Check sheet for the modelled part. Datum: model origin and axes. Units: mm. Face numbers are marked on the shaded views. A direction names the side the tool comes from. Round coordinates to 2 decimals unless told otherwise and drop trailing zeros. Write each loop counter-clockwise with the first axis right and the second up, starting at its lowest first coordinate (ties: lowest second). Pieces come first, ordered by that corner, then holes. Notation, with made-up numbers: M 33,77 L 67,77 A18 ccw 67,102 Z; hole C 54.25,74 d1. An arc over 180 degrees is marked long. Answer in a Markdown table with one row per item.
```python
from build123d import *

# Parameters (mm, degrees)
BOSS_EXTRUDE1_DEPTH     = 9
SHELL1_T                = -1
BOSS_EXTRUDE2_DEPTH     = 2
SKETCH3_R               = 6.5
BOSS_EXTRUDE3_DEPTH     = 1.25
SKETCH4_R               = 5
BOSS_EXTRUDE4_DEPTH     = 0.6
CUT_EXTRUDE1_DEPTH      = 26.78996898
CUT_EXTRUDE1_DEPTH_BACK = 26.78996898
SKETCH5_R               = 3.1
BOSS_EXTRUDE5_DEPTH     = 1.8
SKETCH7_W               = 18.24
SKETCH7_H               = 6.5
BOSS_EXTRUDE6_DEPTH     = 2.5
CUT_EXTRUDE2_REACH      = 31.955
SKETCH8_R               = 2.25
FILLET2_R               = 1
CUT_EXTRUDE3_DEPTH      = 30.432125306
CUT_EXTRUDE3_DEPTH_BACK = 1
SKETCH9_R               = 9


with BuildPart() as part:
    # Sketch1 → Boss-Extrude1 (new body)
    with BuildSketch(Plane(origin=(0, 0, 0), x_dir=(1, 0, 0), z_dir=(0, 1, 0))):
        with BuildLine():
            Line((-9.12, 20), (9.12, 20))
            ThreePointArc((9.12, 20), (9.742253967, 19.742253967), (10, 19.12))
            Line((10, 19.12), (10, -19.12))
            ThreePointArc((10, -19.12), (9.742253967, -19.742253967), (9.12, -20))
            Line((9.12, -20), (-9.12, -20))
            ThreePointArc((-9.12, -20), (-9.742253967, -19.742253967), (-10, -19.12))
            Line((-10, -19.12), (-10, 19.12))
            ThreePointArc((-10, 19.12), (-9.742253967, 19.742253967), (-9.12, 20))
        make_face()
    extrude(amount=BOSS_EXTRUDE1_DEPTH)

    # Shell1
    shell1_openings = [part.faces().sort_by_distance(p)[0] for p in [
        (0, 0, 0),
    ]]
    offset(amount=SHELL1_T, openings=shell1_openings, kind=Kind.INTERSECTION)

    # Sketch2 → Boss-Extrude2 (add)
    with BuildSketch(Plane(origin=(0, 9, 0), x_dir=(1, 0, 0), z_dir=(0, 1, 0))):
        with BuildLine():
            Line((9.5, -14), (-9.5, -14))
            Line((-9.5, -14), (-9.5, 6.877501001))
            ThreePointArc((-9.5, 6.877501001), (0, 20), (9.5, 6.877501001))
            Line((9.5, 6.877501001), (9.5, -14))
        make_face()
    extrude(amount=BOSS_EXTRUDE2_DEPTH)

    # Sketch3 → Boss-Extrude3 (add)
    with BuildSketch(Plane(origin=(0, 11, 0), x_dir=(1, 0, 0), z_dir=(0, 1, 0))):
        with Locations(Location((0, 10, 0), (0, 0, 270))):
            Circle(SKETCH3_R)
    extrude(amount=BOSS_EXTRUDE3_DEPTH)

    # Sketch4 → Boss-Extrude4 (add)
    with BuildSketch(Plane(origin=(0, 12.25, 0), x_dir=(1, 0, 0), z_dir=(0, 1, 0))):
        with Locations(Location((0, 10, 0), (0, 0, 270))):
            Circle(SKETCH4_R)
    extrude(amount=BOSS_EXTRUDE4_DEPTH)

    # Sketch5 → Cut-Extrude1 (cut, two sides: drawn at the far end of the back side and taken through both)
    with BuildSketch(Plane(origin=(0, 12.85, 0), x_dir=(1, 0, 0), z_dir=(0, 1, 0)).offset(-CUT_EXTRUDE1_DEPTH_BACK)):
        with Locations(Location((0, 10, 0), (0, 0, 270))):
            Circle(SKETCH5_R)
    extrude(amount=CUT_EXTRUDE1_DEPTH + CUT_EXTRUDE1_DEPTH_BACK, mode=Mode.SUBTRACT)

    # Sketch6 → Boss-Extrude5 (add)
    with BuildSketch(Plane(origin=(0, 9, 0), x_dir=(1, 0, 0), z_dir=(0, 1, 0))):
        with BuildLine():
            Line((-4.5, -14), (4.5, -14))
            ThreePointArc((4.5, -14), (0, -15.863961031), (-4.5, -14))
        make_face()
    extrude(amount=BOSS_EXTRUDE5_DEPTH)

    # Sketch7 → Boss-Extrude6 (add)
    with BuildSketch(Plane(origin=(0, 0.6, 0), x_dir=(1, 0, 0), z_dir=(0, 1, 0))):
        with Locations((0, 23.25)):
            Rectangle(SKETCH7_W, SKETCH7_H)
        with Locations((0, -23.25)):
            Rectangle(SKETCH7_W, SKETCH7_H)
    extrude(amount=BOSS_EXTRUDE6_DEPTH)

    # Sketch8 → Cut-Extrude2 (cut, up to next)
    with BuildSketch(Plane(origin=(0, 3.1, 0), x_dir=(1, 0, 0), z_dir=(0, 1, 0)), mode=Mode.PRIVATE) as cut_extrude2_sk1:
        with Locations((-4.87, 24.35)):
            Circle(SKETCH8_R)
    cut_extrude2_tool1 = extrude(cut_extrude2_sk1.sketch, amount=-CUT_EXTRUDE2_REACH, mode=Mode.PRIVATE) & part.part
    # Sketch8 → Cut-Extrude2 (cut, up to next)
    with BuildSketch(Plane(origin=(0, 3.1, 0), x_dir=(1, 0, 0), z_dir=(0, 1, 0)), mode=Mode.PRIVATE) as cut_extrude2_sk2:
        with Locations((4.87, 24.35)):
            Circle(SKETCH8_R)
    cut_extrude2_tool2 = extrude(cut_extrude2_sk2.sketch, amount=-CUT_EXTRUDE2_REACH, mode=Mode.PRIVATE) & part.part
    # Sketch8 → Cut-Extrude2 (cut, up to next)
    with BuildSketch(Plane(origin=(0, 3.1, 0), x_dir=(1, 0, 0), z_dir=(0, 1, 0)), mode=Mode.PRIVATE) as cut_extrude2_sk3:
        with Locations((-4.87, -24.35)):
            Circle(SKETCH8_R)
    cut_extrude2_tool3 = extrude(cut_extrude2_sk3.sketch, amount=-CUT_EXTRUDE2_REACH, mode=Mode.PRIVATE) & part.part
    # Sketch8 → Cut-Extrude2 (cut, up to next)
    with BuildSketch(Plane(origin=(0, 3.1, 0), x_dir=(1, 0, 0), z_dir=(0, 1, 0)), mode=Mode.PRIVATE) as cut_extrude2_sk4:
        with Locations((4.87, -24.35)):
            Circle(SKETCH8_R)
    cut_extrude2_tool4 = extrude(cut_extrude2_sk4.sketch, amount=-CUT_EXTRUDE2_REACH, mode=Mode.PRIVATE) & part.part
    add(cut_extrude2_tool1.solids().sort_by_distance((-4.87, 3.1, -24.35))[0], mode=Mode.SUBTRACT)
    add(cut_extrude2_tool2.solids().sort_by_distance((4.87, 3.1, -24.35))[0], mode=Mode.SUBTRACT)
    add(cut_extrude2_tool3.solids().sort_by_distance((-4.87, 3.1, 24.35))[0], mode=Mode.SUBTRACT)
    add(cut_extrude2_tool4.solids().sort_by_distance((4.87, 3.1, 24.35))[0], mode=Mode.SUBTRACT)

    # Fillet2
    fillet2_edges = [part.edges().sort_by_distance(p)[0] for p in [
        (9.12, 1.85, -26.5),
        (-9.12, 1.85, -26.5),
        (-9.12, 1.85, 26.5),
        (9.12, 1.85, 26.5),
    ]]
    fillet(fillet2_edges, radius=FILLET2_R)

    # Sketch9 → Cut-Extrude3 (cut, two sides: drawn at the far end of the back side and taken through both)
    with BuildSketch(Plane.XZ.offset(-8).offset(-CUT_EXTRUDE3_DEPTH_BACK)):
        with Locations(Location((0, -10, 0), (0, 0, 270))):
            Circle(SKETCH9_R)
    extrude(amount=CUT_EXTRUDE3_DEPTH + CUT_EXTRUDE3_DEPTH_BACK, mode=Mode.SUBTRACT)


solid = part.part
```
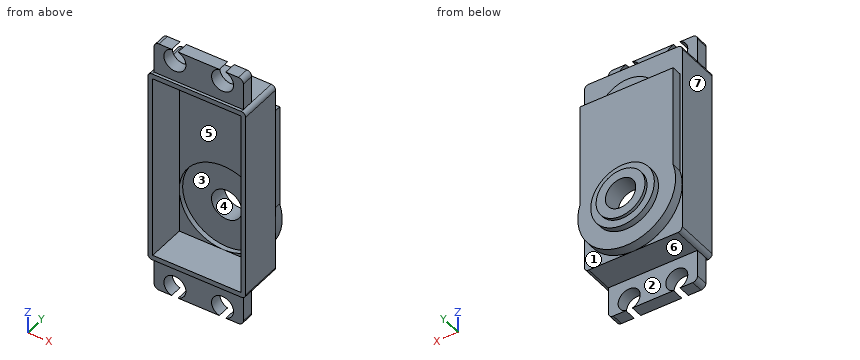
1. Draft check along Z on the marked faces 4, 5, 6 and 7. Enter one of: +Z half, -Z half, draft (parallel to the pull), parting line (faces both ways), or undercut.
Found:
| item | result |
|---|---|
| face 4 | undercut |
| face 5 | undercut |
| face 6 | -Z half |
| face 7 | draft |
2. Section check D-D, the plane y = 6.5. Record the cut outline in (x, z), and give its area (3 significant figures).
Found:
| item | result |
|---|---|
| outline | M -10,-19.12 A0.88 ccw -9.12,-20 L 9.12,-20 A0.88 ccw 10,-19.12 L 10,19.12 A0.88 ccw 9.12,20 L -9.12,20 A0.88 ccw -10,19.12 Z; hole M -9,-19 L 9,-19 L 9,19 L -9,19 Z |
| area | 115 mm2 |
3. Go/stop test with flat-tipped pins: pin 1 (1 mm diameter, centred on y = 10, z = -0.5, fed in from -X); pin 2 (2 mm diameter, centred on y = 2.5, z = -22.5, fed in from -X); pin 3 (1 mm diameter, centred on x = -3.5, y = 10, fed in from +Z). Record where each tip stops, or that it passes through.
Found:
| item | result |
|---|---|
| pin 1 | stops at x = -9.5 |
| pin 2 | stops at x = -9.12 |
| pin 3 | stops at z = 15.11 |
4. Scan lines: L1, parallel to X at y = 1.2, z = -24.35; L2, parallel to X at y = 2.5, z = -8.5; L3, parallel to Z at x = 7.75, y = 7.25. Record each from-to range of solid material in increasing order.
Found:
| item | result |
|---|---|
| L1 | x = -9.12 to -7.12, -2.62 to 2.62, 7.12 to 9.12 |
| L2 | x = -10 to -9, 9 to 10 |
| L3 | z = -20 to -19, 19 to 20 |
5. Section check A-A, the plane y = 9.5. Record the cut outline in (x, z), and give its area (3 significant figures).
Found:
| item | result |
|---|---|
| outline | M -9.5,-6.88 A10 ccw long 9.5,-6.88 L 9.5,14 L 4.5,14 A6.36 ccw -4.5,14 L -9.5,14 Z; hole C 0,-10 d6.2 |
| area | 597 mm2 |
6. Section check B-B, the plane z = -24.35. Record the cut outline in (x, y), and give its area (3 significant figures).
Found:
| item | result |
|---|---|
| outline | M -9.12,0.6 L -7.12,0.6 L -7.12,3.1 L -9.12,3.1 Z; M -2.62,0.6 L 2.62,0.6 L 2.62,3.1 L -2.62,3.1 Z; M 7.12,0.6 L 9.12,0.6 L 9.12,3.1 L 7.12,3.1 Z |
| area | 23.1 mm2 |
7. Access from +Z, -Z, +X, -X, +Y, -Y to the whole of each face (thin tool, end or side, straight path). Record for the marked faces 1, 2 and 3.
Found:
| item | result |
|---|---|
| face 1 | -Z, +X, +Y |
| face 2 | -Z, +X, -X, +Y |
| face 3 | -Y |
8. Section check C-C, the plane z = -12. Record the cut outline in (x, y), and give its area (3 significant figures).
Found:
| item | result |
|---|---|
| outline | M -10,0 L -9,0 L -9,8 L -8.77,8 L -8.77,9 L -2.37,9 L -2.37,12.85 L -4.58,12.85 L -4.58,12.25 L -6.18,12.25 L -6.18,11 L -9.8,11 L -9.8,9 L -10,9 Z; M 2.37,9 L 8.77,9 L 8.77,8 L 9,8 L 9,0 L 10,0 L 10,9 L 9.8,9 L 9.8,11 L 6.18,11 L 6.18,12.25 L 4.58,12.25 L 4.58,12.85 L 2.37,12.85 Z |
| area | 60.4 mm2 |
